```python
from build123d import *

# Parameters (mm, degrees)
PAD005_DEPTH    = 9
POCKET002_DEPTH = 4
CHAMFER002_SIZE = 0.8
POCKET008_DEPTH = 3
CHAMFER007_SIZE = 1.75
CHAMFER008_SIZE = 8.99
POCKET013_DEPTH = 8.001


with BuildPart() as part:
    # Sketch008 → Pad005 (new body)
    with BuildSketch(Plane(origin=(0, 0, 249.45), x_dir=(1, 0, 0), z_dir=(0, -1, 0))):
        Polygon((0.989949, -221.802125), (27.647875, -248.460051), (27.647875, -251.05), (6.76188, -251.05), (-1.6, -242.68812), (-1.6, -221.802125), align=None)
    extrude(amount=PAD005_DEPTH)

    # Sketch009 (on Face7 of Pad005) → Pocket002 (cut)
    with BuildSketch(Plane(origin=(0, 0, 0), x_dir=(1, 0, 0), z_dir=(0, 1, 0))):
        Polygon((22.132442, 0), (18.031223, -4.101219), (13.930004, 0), align=None)
        Polygon((0, -22.132442), (0, -13.930004), (4.101219, -18.031223), align=None)
    extrude(amount=-POCKET002_DEPTH, mode=Mode.SUBTRACT)

    # Chamfer002
    chamfer002_edges = [part.edges().sort_by_distance(p)[0] for p in [
        (18.031223, 0, 0),
        (20.081833, 0, 2.05061),
        (15.980613, 0, 2.05061),
        (0, 0, 18.031223),
        (2.05061, 0, 20.081833),
        (2.05061, 0, 15.980613),
    ]]
    chamfer(chamfer002_edges, length=CHAMFER002_SIZE)

    # Sketch050 → Pocket008 (cut)
    with BuildSketch(Plane(origin=(0, 0, 249.45), x_dir=(1, 0, 0), z_dir=(0, -1, 0))):
        Polygon((0, -225.054816), (2.12132, -222.933496), (26.516504, -247.32868), (24.395184, -249.45), align=None)
    extrude(amount=POCKET008_DEPTH, mode=Mode.SUBTRACT)

    # Chamfer007
    chamfer007_edges = [part.edges().sort_by_distance(p)[0] for p in [
        (17.204877, -9, -1.6),
        (27.647875, -9, -0.305025),
        (14.318912, -9, 14.318912),
        (-1.6, -9, 17.204877),
        (-0.305025, -9, 27.647875),
    ]]
    chamfer(chamfer007_edges, length=CHAMFER007_SIZE)

    # Chamfer008
    chamfer008_edges = [part.edges().sort_by_distance(p)[0] for p in [
        (2.58094, -9, 2.58094),
    ]]
    chamfer(chamfer008_edges, length=CHAMFER008_SIZE)

    # Sketch059 (on Face4 of Chamfer008) → Pocket013 (cut, through all)
    with BuildSketch(Plane(origin=(0, -1, 0), x_dir=(1, 0, 0), z_dir=(0, 1, 0))):
        Polygon((12.643069, -5.23259), (5.23259, -12.643069), (-2.177889, -5.23259), (5.23259, 2.177889), align=None)
    extrude(amount=-POCKET013_DEPTH, mode=Mode.SUBTRACT)


with BuildPart() as part_1:
    # Body001 placement: moved
    add(part.part.moved(Location((0, -249.45, 0))))


solid = part_1.part
```
Geometry check sheet. Reference: the model listing, model coordinates, mm. A direction names the side the tool comes from. Coordinates: 2 decimals unless noted, no trailing zeros. Loops run counter-clockwise (first coordinate to the right, second up) from the corner with the lowest first, then second, coordinate; pieces in that order, holes last. Notation, with made-up numbers: (-38.75, 40) - (-17.75, 40) arc R13 ccw to (-17.75, 54) - close; hole circle Ø7 at (-12, 2.5). An arc over 180 degrees is marked (long way). One line per item, written item: value. Start each with the question number.
(1) Depth check by flat-ended pin: P1, Ø2, axis at x = 19.5, z = 2, coming from the +Y side; P2, Ø6, axis at x = 4.5, z = 2, coming from the -Y side; P3, Ø1.6, axis at x = 17, y = -251.5, coming from the +Z side; P4, Ø10.5, axis at x = 7, z = 7, coming from the -Y side. Enter the tip coordinate at first touch or a pass-through.
(2) Tool access check on faces 5 (the flat face through (27.648, -253, 0)), 6 (the flat face through (16.01, -251.83, 2.08)). Record the directions out of +Z, -Z, +X, -X, +Y, -Y that give a thin tool (end or side, any length) a straight path to the whole face; none if there is none.
(3) Cross-section at D-D on y = -255. Enter the section's corners in (x, z).
(4) Cross-section at A-A on y = -251.75. Enter the section's corners in (x, z).
(5) Material ranges on line 1 (Z direction, x = 19.5, y = -252.5); line 2 (Z direction, x = 18.75, y = -250.5); line 3 (Y direction, x = 5.25, z = 12), recorded low to high. Write a range as [from, to].
(6) Mould release check, pull along Z, two halves, no side actions. Record for faces 1 (the flat face through (-0.04, -257.39, 26.96)), 2 (the flat face through (22.4, -257.6, -0.7)), 3 (the flat face through (6, -250.45, 6)), 4 (the flat face through (11, -258.45, 11)): released by +Z, released by -Z, zero draft, split by the parting line, or undercut.
Results below:
1. P1: stops at y = -249.7
1. P2: stops at y = -250.45
1. P3: stops at z = 8.2
1. P4: stops at y = -258.45
2. face 5: +Z, -Z, +X, +Y, -Y
2. face 6: +Y
3. outline: (-1.6, 14.6) - (2.79, 10.2) - (5.23, 12.64) - (12.64, 5.23) - (10.2, 2.79) - (14.6, -1.6) - (27.65, -1.6) - (27.65, 0.99) - (0.99, 27.65) - (-1.6, 27.65) - close
4. outline: (-1.6, 10) - (0.49, 7.91) - (5.23, 12.64) - (12.64, 5.23) - (7.91, 0.49) - (10, -1.6) - (27.65, -1.6) - (27.65, 0.99) - (26.52, 2.12) - (24.4, 0) - (0, 24.4) - (2.12, 26.52) - (0.99, 27.65) - (-1.6, 27.65) - close; hole (0, 13.93) - (4.1, 18.03) - (0, 22.13) - close; hole (13.93, 0) - (22.13, 0) - (18.03, 4.1) - close
5. line 1: z = [-1.6, 0], [2.63, 9.14]
5. line 2: z = [-1.6, 0], [3.38, 5.65]
5. line 3: y = [-250.45, -249.45]
6. face 1: released by +Z
6. face 2: released by -Z
6. face 3: undercut
6. face 4: zero draft
